from build123d import *

# Parameters (mm, degrees)
SKETCH1_R           = 2
BOSS_EXTRUDE3_DEPTH = 5
FILLET11_R          = 3
FILLET12_R          = 10
FILLET13_R          = 0.5


with BuildPart() as part:
    # Sketch1 → Boss-Extrude3 (new body)
    with BuildSketch(Plane(origin=(0, 0, 0), x_dir=(1, 0, 0), z_dir=(0, 1, 0))):
        with BuildLine():
            Line((-15.194514721, -20.497190469), (-16.934514721, -20.497190469))
            ThreePointArc((-16.934514721, -20.497190469), (-18.487045158, -20.635059579), (-19.990986096, -21.044352024))
            ThreePointArc((-19.990986096, -21.044352024), (-20.009485456, -22.000591241), (-19.982270663, -22.956622109))
            ThreePointArc((-19.982270663, -22.956622109), (-18.512106636, -23.583403018), (-16.917234096, -23.686447466))
            Line((-16.917234096, -23.686447466), (-15.176510207, -23.503489976))
            ThreePointArc((-15.176510207, -23.503489976), (-14.956675222, -24.936847382), (-14.601778477, -26.342866292))
            ThreePointArc((-14.601778477, -26.342866292), (-14.530483873, -26.571223065), (-14.455618246, -26.798434144))
            Line((-14.455618246, -26.798434144), (-16.120081178, -27.339250934))
            ThreePointArc((-16.120081178, -27.339250934), (-17.530103274, -28.082215528), (-18.614519352, -29.250205455))
            ThreePointArc((-18.614519352, -29.250205455), (-18.242481832, -30.131297816), (-17.828767099, -30.993606221))
            ThreePointArc((-17.828767099, -30.993606221), (-16.230770667, -30.968229498), (-14.731870148, -30.413672187))
            Line((-14.731870148, -30.413672187), (-13.216055258, -29.538516018))
            ThreePointArc((-13.216055258, -29.538516018), (-12.432227031, -30.758538224), (-11.536133313, -31.898650905))
            ThreePointArc((-11.536133313, -31.898650905), (-11.378121368, -32.07826709), (-11.217313126, -32.255384164))
            Line((-11.217313126, -32.255384164), (-12.517905671, -33.426442952))
            ThreePointArc((-12.517905671, -33.426442952), (-13.503834046, -34.678682508), (-14.019433156, -36.186766135))
            ThreePointArc((-14.019433156, -36.186766135), (-13.321187423, -36.84036277), (-12.592507783, -37.459847758))
            ThreePointArc((-12.592507783, -37.459847758), (-11.142987043, -36.786701267), (-9.999232057, -35.670430194))
            Line((-9.999232057, -35.670430194), (-8.970424328, -34.254397795))
            ThreePointArc((-8.970424328, -34.254397795), (-7.758133877, -35.050131881), (-6.47578593, -35.727202496))
            ThreePointArc((-6.47578593, -35.727202496), (-6.258378327, -35.827020809), (-6.03943266, -35.923418714))
            Line((-6.03943266, -35.923418714), (-6.751270551, -37.522232796))
            ThreePointArc((-6.751270551, -37.522232796), (-7.142629255, -39.067223735), (-7.000259644, -40.654639727))
            ThreePointArc((-7.000259644, -40.654639727), (-6.096538725, -40.967727841), (-5.178889508, -41.23727483))
            ThreePointArc((-5.178889508, -41.23727483), (-4.128479759, -40.032751715), (-3.537635932, -38.547780286))
            Line((-3.537635932, -38.547780286), (-3.173725562, -36.835716518))
            ThreePointArc((-3.173725562, -36.835716518), (-1.742588917, -37.069572835), (-0.295716346, -37.166529725))
            ThreePointArc((-0.295716346, -37.166529725), (-0.056504827, -37.169290654), (0.182720579, -37.168301296))
            Line((0.182720579, -37.168301296), (0.182720579, -38.918421193))
            ThreePointArc((0.182720579, -38.918421193), (0.453601009, -40.489020569), (1.229322337, -41.881290308))
            ThreePointArc((1.229322337, -41.881290308), (2.182256886, -41.799734123), (3.130205798, -41.672735992))
            ThreePointArc((3.130205798, -41.672735992), (3.59987917, -40.145109238), (3.535649575, -38.548202499))
            Line((3.535649575, -38.548202499), (3.171739177, -36.836138737))
            ThreePointArc((3.171739177, -36.836138737), (15.191099578, -23.357875025), (5.935485279, -7.851030694))
            Line((5.935485279, -7.851030694), (5.935485279, 54.590604732))
            ThreePointArc((5.935485279, 54.590604732), (-0.947505363, 71.20761409), (-17.564514721, 78.090604732))
            Line((-17.564514721, 78.090604732), (-17.564514721, 68.090604732))
            ThreePointArc((-17.564514721, 68.090604732), (-8.018573175, 64.136546278), (-4.064514721, 54.590604732))
            Line((-4.064514721, 54.590604732), (-4.064514721, -7.200645488))
            ThreePointArc((-4.064514721, -7.200645488), (-11.701584545, -12.114472137), (-15.194514721, -20.497190469))
        make_face()
        with Locations((0, -21.909395268)):
            Circle(SKETCH1_R, mode=Mode.SUBTRACT)
        with Locations((-12.564514721, 72.402117863)):
            Circle(SKETCH1_R, mode=Mode.SUBTRACT)
    extrude(amount=BOSS_EXTRUDE3_DEPTH)

    # Fillet11
    fillet11_edges = [part.edges().sort_by_distance(p)[0] for p in [
        (-4.064514721, 2.5, 7.200645488),
        (-17.564514721, 2.5, -68.090604732),
        (-17.564514721, 2.5, -78.090604732),
    ]]
    fillet(fillet11_edges, radius=FILLET11_R)

    # Fillet12
    fillet12_edges = [part.edges().sort_by_distance(p)[0] for p in [
        (5.935485279, 2.5, 7.851030694),
    ]]
    fillet(fillet12_edges, radius=FILLET12_R)

    # Fillet13
    fillet13_edges = [part.edges().sort_by_distance(p)[0] for p in [
        (3.130205798, 2.5, 41.672735992),
        (1.229322337, 2.5, 41.881290308),
        (-5.178889508, 2.5, 41.23727483),
        (-7.000259644, 2.5, 40.654639727),
        (-12.592507783, 2.5, 37.459847758),
        (-14.019433156, 2.5, 36.186766135),
        (-17.828767099, 2.5, 30.993606221),
        (-18.614519352, 2.5, 29.250205455),
        (-19.982270663, 2.5, 22.956622109),
        (-19.990986096, 2.5, 21.044352024),
    ]]
    fillet(fillet13_edges, radius=FILLET13_R)


solid = part.part
CAD build for the part. Positions are in the model's coordinates, mm. A direction names the side the tool comes from. Give positions to 0.01 mm unless a question says otherwise; leave off trailing zeros. Loops run counter-clockwise (first coordinate to the right, second up) from the corner with the lowest first, then second, coordinate; pieces in that order, holes last. Notation, with made-up numbers: M 85.5,17 L 144.5,17 A9 ccw 144.5,21 Z; hole C 60,-38.75 d10. An arc over 180 degrees is marked long. Answer in a Markdown table with one row per item. Add a question column.
Item 1: Mould opens along Z. For faces 1 (the face through (-3, 0, -6)), 2 (the face through (-11.044, 2.465, 36.717)), 3 (the face through (-12.234, 2.465, 12.788)) say: +Z half, -Z half, draft (parallel to the pull), parting line (faces both ways), or undercut.
Item 2: Tool access for faces 4 (the face through (-17.565, 2, -73)), 5 (the face through (-4.58, 2.54, 6.75)), 6 (the face through (-4.067, 2.465, 39.929)), 7 (the face through (5.935, 2, -26)): list every direction of +Z, -Z, +X, -X, +Y, -Y with a clear straight run to the whole face (end or side of a thin tool).
Item 3: Probe probe 1 along Z at (x, y) = (-13.5, 1.15); probe 2 along X at (y, z) = (3.65, -48); probe 3 along Z at (x, y) = (0, 1.1). List the from-to ranges inside material, lowest first.
Item 4: Band-saw the part on C-C on z = 17.5. Give the cut face in (x, y).
Item 5: Band-saw the part on B-B on x = 7.5. Give the cut face in (y, z).
Item 6: Band-saw the part on A-A on y = 1.9. Give the number of separate pieces and of enclosed holes in the cut face, then the cut area to 3 significant figures.
Item 7: Drop flat-ended pins along their axis: P1, Ø2, axis at y = 1, z = -32.5, coming from the +X side; P2, Ø2, axis at y = 1, z = 28.5, coming from the -X side; P3, Ø1, axis at x = -6.5, y = 2.5, coming from the +Z side; P4, Ø1.5, axis at x = -6.5, z = -27, coming from the +Y side. Give the stop position or say it passes through.
Reply:
| question | item | result |
|---|---|---|
| 1 | face 1 | draft |
| 1 | face 2 | +Z half |
| 1 | face 3 | undercut |
| 2 | face 4 | -Z, -X, +Y, -Y |
| 2 | face 5 | -X, +Y, -Y |
| 2 | face 6 | +Z, +Y, -Y |
| 2 | face 7 | -Z, +X, +Y, -Y |
| 3 | probe 1 | z = -77.74 to -74.17, -70.63 to -67.46, 14.79 to 29.7, 34.67 to 36.68 |
| 3 | probe 2 | x = -4.06 to 5.94 |
| 3 | probe 3 | z = -70.2 to 19.91, 23.91 to 37.17 |
| 4 | outline | M -14.61,0 L 14.61,0 L 14.61,5 L -14.61,5 Z |
| 5 | outline | M 0,7.68 L 5,7.68 L 5,35.2 L 0,35.2 Z |
| 6 | separate pieces | 1 |
| 6 | enclosed holes | 2 |
| 6 | area | 1,690 mm^2 |
| 7 | P1 | stops at x = 5.94 |
| 7 | P2 | stops at x = -18.55 |
| 7 | P3 | stops at z = 41 |
| 7 | P4 | passes through |
